from build123d import *

# Parameters (mm, degrees)
BOSS_EXTRUDE1_DEPTH = 25.4
FILLET1_R           = 20.32
SHELL1_T            = -2.54
SKETCH2_R           = 2.54
CUT_EXTRUDE1_DEPTH  = 347.409815103
CUT_EXTRUDE2_DEPTH  = 347.409815103


with BuildPart() as part:
    # Sketch1 → Boss-Extrude1 (new body)
    with BuildSketch(Plane(origin=(0, 0, 0), x_dir=(1, 0, 0), z_dir=(0, 1, 0))):
        Polygon((-279.4, 203.2), (-279.4, -203.2), (279.4, -203.2), (279.4, 203.2), (152.4, 203.2), (152.4, 12.7), (-152.4, 12.7), (-152.4, 203.2), align=None)
    extrude(amount=BOSS_EXTRUDE1_DEPTH)

    # Fillet1
    fillet1_edges = [part.edges().sort_by_distance(p)[0] for p in [
        (279.4, 12.7, -203.2),
        (-279.4, 12.7, -203.2),
        (-152.4, 12.7, -203.2),
        (152.4, 12.7, -203.2),
    ]]
    fillet(fillet1_edges, radius=FILLET1_R)

    # Shell1
    shell1_openings = [part.faces().sort_by_distance(p)[0] for p in [
        (0, 0, 37.577423361),
    ]]
    offset(amount=SHELL1_T, openings=shell1_openings, kind=Kind.INTERSECTION)

    # Sketch2 → Cut-Extrude1 (cut, through all)
    with BuildSketch(Plane(origin=(0, 25.4, 0), x_dir=(1, 0, 0), z_dir=(0, 1, 0))):
        with Locations(Location((-177.72, 165.1, 0), (0, 0, 270))):
            Circle(SKETCH2_R)
        with Locations(Location((-167.56, 165.1, 0), (0, 0, 270))):
            Circle(SKETCH2_R)
        with Locations(Location((167.56, 165.1, 0), (0, 0, 270))):
            Circle(SKETCH2_R)
        with Locations(Location((177.72, 165.1, 0), (0, 0, 270))):
            Circle(SKETCH2_R)
    extrude(amount=-CUT_EXTRUDE1_DEPTH, mode=Mode.SUBTRACT)

    # Sketch3 → Cut-Extrude2 (cut, through all)
    with BuildSketch(Plane(origin=(0, 25.4, 0), x_dir=(1, 0, 0), z_dir=(0, 1, 0))):
        Polygon((279.4, -253.088506779), (279.4, -25.4), (0, -25.4), (0, 203.2), (-296.633483773, 203.2), (-305.626462942, -253.088506779), align=None)
    extrude(amount=-CUT_EXTRUDE2_DEPTH, mode=Mode.SUBTRACT)


solid = part.part
Model file for the job. Use its own axes, mm. A direction names the side the tool comes from. Give positions to 0.01 mm unless a question says otherwise; leave off trailing zeros. Write each loop counter-clockwise with the first axis right and the second up, starting at its lowest first coordinate (ties: lowest second). Pieces come first, ordered by that corner, then holes. Notation, with made-up numbers: M 57,0.5 L 95,0.5 A23 ccw 95,12.5 Z; hole C 83.25,48.25 d8. An arc over 180 degrees is marked long. One line per item, written item: value. Start each with the question number.
Q1. Saw through at C-C, the plane x = 112.5. Write the cut outline in (y, z), plus the area to 3 significant figures.
Q2. Saw through at A-A, the plane z = -152. Write the cut outline in (x, y), plus the area to 3 significant figures.
Q3. Probe probe 1 along X at (y, z) = (23.6, -165.1); probe 2 along X at (y, z) = (9.25, -104); probe 3 along Z at (x, y) = (27.5, 15.75). List the from-to ranges inside material, lowest first. Write a range as [from, to].
Q4. Two-plate mould, pull along X, no slides. Class faces 4 (the cylindrical face through (271.79, 11.59, -195.313)), 5 (the flat face through (217, 13, -203.2)), 6 (the flat face through (152.4, 13, -99)): +X half, -X half, draft (parallel to the pull), parting line (faces both ways), or undercut.
Q5. Saw through at D-D, the plane x = 193.5. Write the cut outline in (y, z).
Q6. Saw through at B-B, the plane y = 7.5. Write the cut outline in (x, z), plus the area to 3 significant figures.
Q7. 3-axis set-ups, long thin cutter, end or side, ignore diameter. For faces 1 (the flat face through (77, 13, -12.7)), 2 (the flat face through (217, 11, -200.66)), 3 (the flat face through (79, 11, -10.16)): which of +Z, -Z, +X, -X, +Y, -Y reach the whole face in a straight line?
Q8. Drop flat-ended pins along their axis: pin 1 Ø6 at (y, z) = (18, -155) entering from -X; pin 2 Ø4 at (x, y) = (154, 10) entering from -Z; pin 3 Ø1 at (x, y) = (239, 8.5) entering from +Z. Give the stop position or say it passes through.
Output values:
1. outline: M 0,-12.7 L 25.4,-12.7 L 25.4,25.4 L 22.86,25.4 L 22.86,-10.16 L 0,-10.16 Z
1. area: 155 mm²
2. outline: M 152.4,0 L 154.94,0 L 154.94,22.86 L 276.86,22.86 L 276.86,0 L 279.4,0 L 279.4,25.4 L 152.4,25.4 Z
2. area: 439 mm²
3. probe 1: x = [152.4, 165.02], [170.1, 175.18], [180.26, 279.4]
3. probe 2: x = [152.4, 154.94], [276.86, 279.4]
3. probe 3: z = [-12.7, -10.16]
4. face 4: undercut
4. face 5: draft
4. face 6: -X half
5. outline: M 0,-203.2 L 25.4,-203.2 L 25.4,25.4 L 22.86,25.4 L 22.86,-200.66 L 0,-200.66 Z
6. outline: M 0,-12.7 L 152.4,-12.7 L 152.4,-182.88 A20.32 ccw 172.72,-203.2 L 259.08,-203.2 A20.32 ccw 279.4,-182.88 L 279.4,25.4 L 276.86,25.4 L 276.86,-182.88 A17.78 cw 259.08,-200.66 L 172.72,-200.66 A17.78 cw 154.94,-182.88 L 154.94,-10.16 L 0,-10.16 Z
6. area: 1,730 mm²
7. face 1: -Z, -X, +Y, -Y
7. face 2: +Z, -Y
7. face 3: +Z, -X, -Y
8. pin 1: stops at x = 152.4
8. pin 2: stops at z = -194.43
8. pin 3: stops at z = -200.66
